from build123d import *

# Parameters (mm, degrees)
F0_W     = 1500
F0_H     = 150
F0_R     = 30
F1_DEPTH = 50
F2_R     = 50


with BuildPart() as f1:
    # F0 (on Front) → F1 (new body)
    with BuildSketch(Plane.XZ):
        with Locations((275.430977, 356.40495)):
            Rectangle(F0_W, F0_H)
        with Locations((-424.569023, 356.40495)):
            Circle(F0_R, mode=Mode.SUBTRACT)
        with Locations((275.430977, 356.40495)):
            Circle(F0_R, mode=Mode.SUBTRACT)
        with Locations((975.430977, 356.40495)):
            Circle(F0_R, mode=Mode.SUBTRACT)
    extrude(amount=F1_DEPTH)

    # F2
    f2_edges = [f1.edges().sort_by_distance(p)[0] for p in [
        (-474.569023, -25, 431.40495),
        (-474.569023, -25, 281.40495),
        (1025.430977, -25, 431.40495),
        (1025.430977, -25, 281.40495),
    ]]
    fillet(f2_edges, radius=F2_R)


solid = f1.part
The model under review builds one solid part; all positions refer to its coordinate system, in mm. Round coordinates to 2 decimals unless told otherwise and drop trailing zeros. Write each loop counter-clockwise with the first axis right and the second up, starting at its lowest first coordinate (ties: lowest second). Pieces come first, ordered by that corner, then holes. Notation, with made-up numbers: (14.25, -17) - (49.25, -17) arc R22 cw to (49.25, 15) - close; hole circle Ø3 at (19, 22.25). An arc over 180 degrees is marked (long way). One line per item, written item: value. Start each with the question number.
1. The part is to be moulded in two halves that separate along X. For faces 1 (the face through (-460.31, -25.35, 416.37)), 2 (the face through (268.928, -24.65, 327.118)), 3 (the face through (1010.395, -25.35, 417.147)), 4 (the face through (265, 0, 324)), say which applies: released by +X, released by -X, zero draft, split by the parting line, or undercut.
2. Consider section B-B on z = 413.5. Write out the cut boundary in (x, y).
3. Clearance check with flat-ended pins moving along their axes: P1, Ø6, axis at y = -20.5, z = 324, coming from the +X side; P2, Ø8, axis at y = -31, z = 314.5, coming from the -X side; P3, Ø3, axis at x = 132, z = 352, coming from the +Y side; P4, Ø8, axis at y = -41, z = 391.5, coming from the -X side. State where each tip first meets the part, or that it passes through.
4. To check wall thickness, follow L1, parallel to X at y = -32.5, z = 364; L2, parallel to X at y = -36, z = 376; L3, parallel to Z at x = 299, y = -16.5. State the ranges of each line that lie inside material, in increasing order. Write a range as from..to.
5. Consider section A-A on y = -25. Write out the cut boundary in (x, z).
Checks:
1. face 1: released by -X
1. face 2: undercut
1. face 3: released by +X
1. face 4: zero draft
2. outline: (-462.91, -50) - (1013.77, -50) - (1013.77, 0) - (-462.91, 0) - close
3. P1: stops at x = 1025.24
3. P2: stops at x = -472.87
3. P3: stops at y = 0
3. P4: stops at x = -474.2
4. L1: x = -474.57..-453.59, -395.55..246.41, 304.45..946.41, 1004.45..1025.43
4. L2: x = -474.57..-447.29, -401.85..252.71, 298.15..952.71, 998.15..1025.43
4. L3: z = 281.4..337.84, 374.97..431.4
5. outline: (-474.57, 331.4) arc R50 ccw to (-424.57, 281.4) - (975.43, 281.4) arc R50 ccw to (1025.43, 331.4) - (1025.43, 381.4) arc R50 ccw to (975.43, 431.4) - (-424.57, 431.4) arc R50 ccw to (-474.57, 381.4) - close; hole circle Ø60 at (-424.57, 356.4); hole circle Ø60 at (275.43, 356.4); hole circle Ø60 at (975.43, 356.4)
